Job drawing, mm, ordinate dimensions from the low corner. One solid piece. A direction names the side the tool comes from. Round coordinates to 2 decimals unless told otherwise and drop trailing zeros. Loops run counter-clockwise (first coordinate to the right, second up) from the corner with the lowest first, then second, coordinate; pieces in that order, holes last.
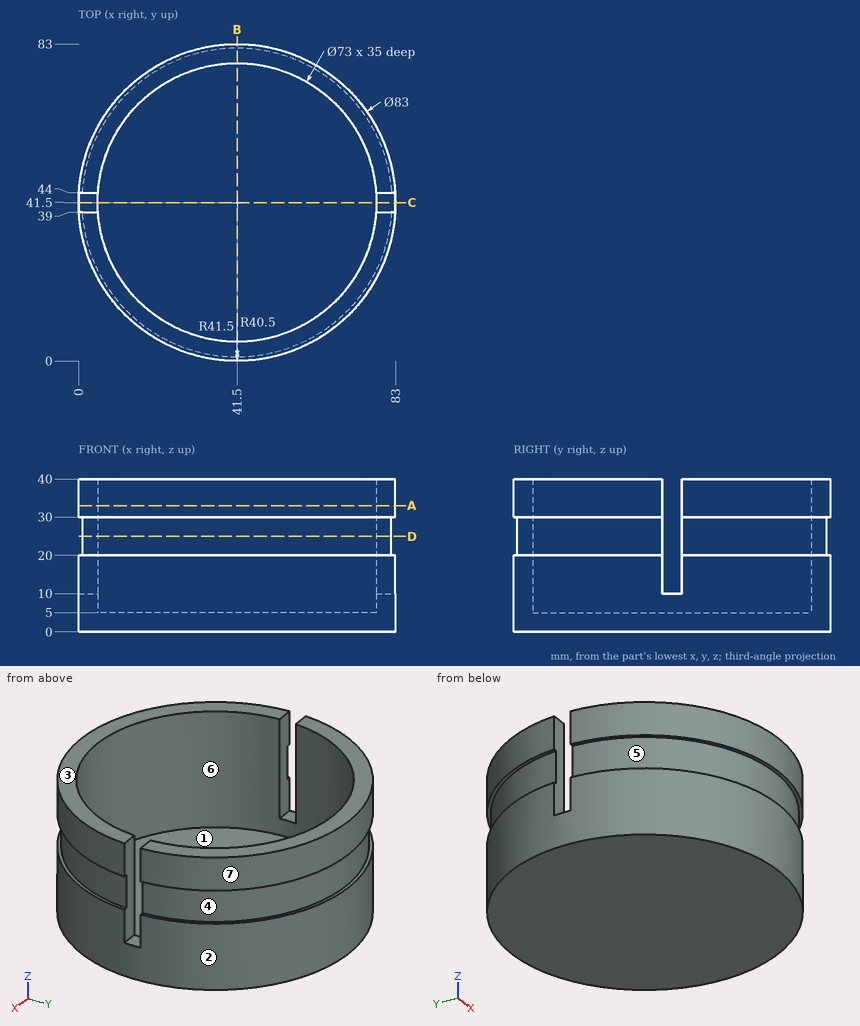
Item 1: Cut at C-C, the plane y = 41.5. Give the cut face in (x, z).
Answers follow:
outline: (0, 0) - (83, 0) - (83, 10) - (78, 10) - (78, 5) - (5, 5) - (5, 10) - (0, 10) - close
Item 2: 3-axis set-ups, long thin cutter, end or side, ignore diameter. For the marked faces 4, 5, 6 and 7: which of +Z, -Z, +X, -X, +Y, -Y reach the whole face in a straight line?
Answers follow:
face 4: +Y
face 5: -Y
face 6: +Z
face 7: +Z, -Z, +Y
Item 3: Flat gauge pins, fed straight in: P1, Ø1, axis at y = 15.5, z = 9, coming from the -X side; P2, Ø2, axis at x = 58.5, z = 13, coming from the -Y side; P3, Ø19.5, axis at x = 49.5, y = 21, coming from the +Z side. Where does each tip first touch, or does it go through?
Answers follow:
P1: stops at x = 8.76
P2: stops at y = 3.21
P3: stops at z = 5
Item 4: Cut at A-A, the plane z = 33. Give the cut face in (x, y), plus the area to 3 significant figures.
Answers follow:
outline: (0.08, 39) arc R41.5 ccw to (82.92, 39) - (77.91, 39) arc R36.5 cw to (5.09, 39) - close; (0.08, 44) - (5.09, 44) arc R36.5 cw to (77.91, 44) - (82.92, 44) arc R41.5 ccw to start
area: 1,180 mm2
Item 5: Probe line 1 (Y direction, x = 42, z = 27); line 2 (Y direction, x = 41.5, z = 13.5); line 3 (Z direction, x = 47, y = 55). List the from-to ranges inside material, lowest first.
Answers follow:
line 1: y = 1 to 5, 78 to 82
line 2: y = 0 to 5, 78 to 83
line 3: z = 0 to 5
Item 6: Cut at D-D, the plane z = 25. Give the cut face in (x, y), plus the area to 3 significant figures.
Answers follow:
outline: (1.08, 39) arc R40.5 ccw to (81.92, 39) - (77.91, 39) arc R36.5 cw to (5.09, 39) - close; (1.08, 44) - (5.09, 44) arc R36.5 cw to (77.91, 44) - (81.92, 44) arc R40.5 ccw to start
area: 928 mm2
Item 7: Cut at B-B, the plane x = 41.5. Give the cut face in (y, z), plus the area to 3 significant figures.
Answers follow:
outline: (0, 0) - (83, 0) - (83, 20) - (82, 20) - (82, 30) - (83, 30) - (83, 40) - (78, 40) - (78, 5) - (5, 5) - (5, 40) - (0, 40) - (0, 30) - (1, 30) - (1, 20) - (0, 20) - close
area: 745 mm2
Item 8: Two-plate mould, pull along Y, no slides. Class the marked faces 1, 2 and 3: released by +Y, released by -Y, zero draft, split by the parting line, or undercut.
Answers follow:
face 1: undercut
face 2: split by the parting line
face 3: zero draft
